Verification items for the finished model (mm, model axes). A direction names the side the tool comes from. Give positions to 0.01 mm unless a question says otherwise; leave off trailing zeros. Order: outer loops, then holes, each group sorted by start corner. A loop starts at its lowest first (then second) coordinate and runs counter-clockwise, first axis right, second up. Notation, with made-up numbers: (21, -28) - (32, -28) arc R35 cw to (32, 10) - close; hole circle Ø3 at (-11.5, 10.25). An arc over 180 degrees is marked (long way). Answer as a JSON object with one key per item and string values.
```python
from build123d import *

# Parameters (mm, degrees)
SKETCH_1_R          = 5
EXTRUDE_1_DEPTH     = 5
SKETCH_2_W          = 10
SKETCH_2_H          = 6
EXTRUDE_2_DEPTH     = 5
SKETCH_3_R          = 1.25
CUT_EXTRUDE_2_DEPTH = 150.485785277


with BuildPart() as part:
    # Эскиз1 → Бобышка-Вытянуть1 (new body)
    with BuildSketch(Plane(origin=(0, 0, 0), x_dir=(0, 0, -1), z_dir=(1, 0, 0))):
        with BuildLine():
            Line((0, 0), (39.5, 0))
            Line((39.5, 0), (39.5, 9))
            ThreePointArc((39.5, 9), (49.5, 19), (59.5, 9))
            Line((59.5, 9), (59.5, 0))
            Line((59.5, 0), (85.5, 0))
            Line((85.5, 0), (85.5, 9))
            ThreePointArc((85.5, 9), (95.5, 19), (105.5, 9))
            Line((105.5, 9), (105.5, 0))
            Line((105.5, 0), (145, 0))
            Line((145, 0), (145, 30))
            Line((145, 30), (0, 30))
            Line((0, 30), (0, 0))
        make_face()
        with Locations((27.5, 21)):
            Circle(SKETCH_1_R, mode=Mode.SUBTRACT)
        with Locations((72.5, 21)):
            Circle(SKETCH_1_R, mode=Mode.SUBTRACT)
        with Locations((117.5, 21)):
            Circle(SKETCH_1_R, mode=Mode.SUBTRACT)
    extrude(amount=EXTRUDE_1_DEPTH)

    # Эскиз2 → Бобышка-Вытянуть2 (add)
    with BuildSketch(Plane(origin=(5, 0, 0), x_dir=(0, 0, -1), z_dir=(1, 0, 0))):
        with Locations((5, 33)):
            Rectangle(SKETCH_2_W, SKETCH_2_H)
        with Locations((50, 33)):
            Rectangle(SKETCH_2_W, SKETCH_2_H)
        with Locations((95, 33)):
            Rectangle(SKETCH_2_W, SKETCH_2_H)
        with Locations((140, 33)):
            Rectangle(SKETCH_2_W, SKETCH_2_H)
    extrude(amount=-EXTRUDE_2_DEPTH)

    # Эскиз3 → Вырез-Вытянуть2 (cut, through all)
    with BuildSketch(Plane.XY):
        with BuildLine():
            Line((0, 36), (0, 33.5))
            ThreePointArc((0, 33.5), (0.732233047, 35.267766953), (2.5, 36))
            Line((2.5, 36), (0, 36))
        make_face()
        with BuildLine():
            ThreePointArc((2.5, 36), (4.267766953, 35.267766953), (5, 33.5))
            Line((5, 33.5), (5, 36))
            Line((5, 36), (2.5, 36))
        make_face()
        with Locations((2.5, 33.5)):
            Circle(SKETCH_3_R)
    extrude(amount=-CUT_EXTRUDE_2_DEPTH, mode=Mode.SUBTRACT)


solid = part.part
```
(1) Section check C-C (y = 14). Record the cut outline in (x, z).
Computed values:
{"outline": "(0, -145) - (5, -145) - (5, -104.16) - (0, -104.16) - close; (0, -86.84) - (5, -86.84) - (5, -58.16) - (0, -58.16) - close; (0, -40.84) - (5, -40.84) - (5, 0) - (0, 0) - close"}
(2) Release check for a two-part mould opening along X. For faces 4 (the cylindrical face through (3.077, 32.391, -4.93)), 5 (the flat face through (5, 13, -71)), 6 (the flat face through (2, 4, -85.5)) record: pulls with the +X half, pulls with the -X half, needs draft (parallel to the pull), parting line crosses it, or undercut.
Computed values:
{"face 4": "undercut", "face 5": "pulls with the +X half", "face 6": "needs draft"}
(3) Gauge pin test, flat ends, axial feed: pin 1 Ø1.5 at (x, z) = (1.5, -55.5) entering from -Y; pin 2 Ø1 at (x, z) = (4, -76.5) entering from +Y. Record the tip position at first contact, or that the pin passes through.
Computed values:
{"pin 1": "stops at y = 16.38", "pin 2": "stops at y = 30"}
(4) Section check B-B (y = 21). Record the cut outline in (x, z).
Computed values:
{"outline": "(0, -145) - (5, -145) - (5, -122.5) - (0, -122.5) - close; (0, -112.5) - (5, -112.5) - (5, -77.5) - (0, -77.5) - close; (0, -67.5) - (5, -67.5) - (5, -32.5) - (0, -32.5) - close; (0, -22.5) - (5, -22.5) - (5, 0) - (0, 0) - close"}
(5) Section check A-A (z = -117.5). Record the cut outline in (x, y).
Computed values:
{"outline": "(0, 0) - (5, 0) - (5, 16) - (0, 16) - close; (0, 26) - (5, 26) - (5, 30) - (0, 30) - close"}
(6) Material ranges on line 1 along Z through (x, y) = (1.1, 21.5); line 2 along Z through (x, y) = (2.95, 7); line 3 along Z through (x, y) = (4.7, 31), recorded low to high. Write a range as [from, to].
Computed values:
{"line 1": "z = [-145, -122.47], [-112.53, -77.47], [-67.53, -32.47], [-22.53, 0]", "line 2": "z = [-145, -105.5], [-85.5, -59.5], [-39.5, 0]", "line 3": "z = [-145, -135], [-100, -90], [-55, -45], [-10, 0]"}
(7) Section check D-D (z = -49.5). Record the cut outline in (x, y).
Computed values:
{"outline": "(0, 19) - (5, 19) - (5, 33.5) arc R2.5 ccw to (0, 33.5) - close; hole circle Ø2.5 at (2.5, 33.5)"}
(8) Access from +Z, -Z, +X, -X, +Y, -Y to the whole of each face (thin tool, end or side, straight path). Record for faces 1 (the cylindrical face through (2.465, 19.085, -122.119)), 2 (the flat face through (2, 4, -39.5)), 3 (the flat face through (3, 32, -135)).
Computed values:
{"face 1": "+X, -X", "face 2": "+X, -X, -Y", "face 3": "+X, -X, +Y"}
